The model under review builds one solid part; all positions refer to its coordinate system, in mm. Give positions to 0.01 mm unless a question says otherwise; leave off trailing zeros. Loops run counter-clockwise (first coordinate to the right, second up) from the corner with the lowest first, then second, coordinate; pieces in that order, holes last. Notation, with made-up numbers: M 81,67 L 137,67 A21 cw 137,101 Z; hole C 67,-10 d1. An arc over 180 degrees is marked long. Write item = value, one per line. Start each with the question number.
1. We need section A-A on y = 83.5. Give the boundary of the cut face in (x, z).
2. Wall thickness on line 1 along Z through (x, y) = (-38.5, 66.5); line 2 along X through (y, z) = (71, -25.5); line 3 along Y through (x, z) = (-40, -27): over which ranges is each line inside the solid? List them lowest first. Write a range as from..to.
3. For pin 1 (2 mm diameter, centred on x = -38, z = -26, fed in from -Y); pin 2 (3.5 mm diameter, centred on x = -39, y = 70, fed in from +Z); pin 3 (1.5 mm diameter, centred on x = -38, z = -24.5, fed in from -Y), all flat-tipped, find the tip position at first contact; note any pin that passes through.
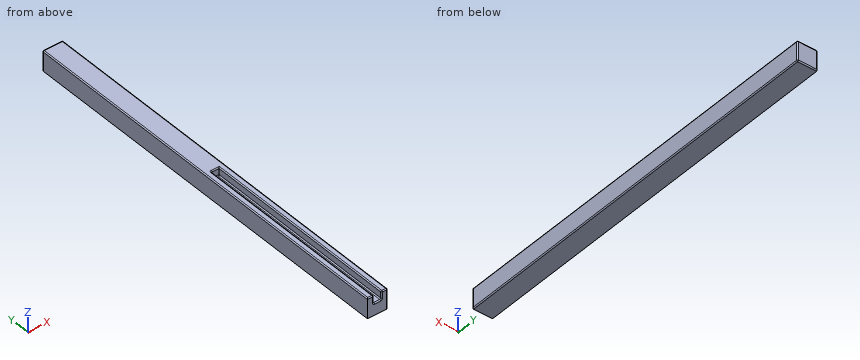
from build123d import *

# Parameters (mm, degrees)
SKETCH1_W           = 10
SKETCH1_H           = 10
BOSS_EXTRUDE1_DEPTH = 200
SKETCH2_W           = 4
SKETCH2_H           = 100
CUT_EXTRUDE1_DEPTH  = 4
FILLET1_R           = 0.5


with BuildPart() as part:
    # Sketch1 → Boss-Extrude1 (new body)
    with BuildSketch(Plane(origin=(0, 0, 0), x_dir=(1, 0, 0), z_dir=(0, 1, 0))):
        with Locations((-38.49189023, 27.694440025)):
            Rectangle(SKETCH1_W, SKETCH1_H)
    extrude(amount=BOSS_EXTRUDE1_DEPTH)

    # Sketch2 → Cut-Extrude1 (cut)
    with BuildSketch(Plane.XY.offset(-22.694440025)):
        with Locations((-38.49189023, 50)):
            Rectangle(SKETCH2_W, SKETCH2_H)
    extrude(amount=-CUT_EXTRUDE1_DEPTH, mode=Mode.SUBTRACT)

    # Fillet1
    fillet1_edges = [part.edges().sort_by_distance(p)[0] for p in [
        (-33.49189023, 200, -27.694440025),
        (-38.49189023, 200, -32.694440025),
        (-34.99189023, 0, -22.694440025),
        (-40.49189023, 50, -26.694440025),
        (-40.49189023, 0, -24.694440025),
        (-38.49189023, 100, -22.694440025),
        (-40.49189023, 100, -24.694440025),
        (-36.49189023, 50, -22.694440025),
        (-38.49189023, 0, -26.694440025),
        (-36.49189023, 0, -24.694440025),
        (-38.49189023, 100, -26.694440025),
        (-36.49189023, 50, -26.694440025),
        (-40.49189023, 50, -22.694440025),
        (-43.49189023, 200, -27.694440025),
        (-33.49189023, 0, -27.694440025),
        (-41.99189023, 0, -22.694440025),
        (-38.49189023, 200, -22.694440025),
        (-33.49189023, 100, -32.694440025),
        (-33.49189023, 100, -22.694440025),
        (-43.49189023, 100, -22.694440025),
    ]]
    fillet(fillet1_edges, radius=FILLET1_R)


solid = part.part
Final values:
q1.outline = M -43.49,-32.69 L -33.99,-32.69 A0.5 ccw -33.49,-32.19 L -33.49,-23.19 A0.5 ccw -33.99,-22.69 L -35.99,-22.69 A0.5 ccw -36.49,-23.19 L -36.49,-26.19 A0.5 cw -36.99,-26.69 L -39.99,-26.69 A0.5 cw -40.49,-26.19 L -40.49,-23.19 A0.5 ccw -40.99,-22.69 L -42.99,-22.69 A0.5 ccw -43.49,-23.19 Z
q2.line_1 = -32.69..-26.69
q2.line_2 = -43.49..-40.49, -36.49..-33.49
q2.line_3 = 0.04..200
q3.pin_1 = 0.04
q3.pin_2 = -22.76
q3.pin_3 = 100
